The model under review builds one solid part; all positions refer to its coordinate system, in mm. Face numbers are marked on the shaded views. A direction names the side the tool comes from. Coordinates: 2 decimals unless noted, no trailing zeros. Write each loop counter-clockwise with the first axis right and the second up, starting at its lowest first coordinate (ties: lowest second). Pieces come first, ordered by that corner, then holes. Notation, with made-up numbers: (42, -26) - (84, -26) arc R18 ccw to (84, 6) - close; hole circle Ø5 at (29, 2). An arc over 180 degrees is marked (long way). Use one line per item in the form item = value. Start each with the question number.
```python
from build123d import *

# Parameters (mm, degrees)
CROQUIS3_W              = 44
CROQUIS3_H              = 60.5
SALIENTE_EXTRUIR1_DEPTH = 2
SALIENTE_EXTRUIR2_DEPTH = 19
CROQUIS5_W              = 3
CROQUIS5_H              = 13
SALIENTE_EXTRUIR3_DEPTH = 5
CROQUIS6_W              = 40
CROQUIS6_H              = 56.5
CROQUIS6_W_2            = 38
CROQUIS6_H_2            = 54.5
CORTAR_EXTRUIR1_DEPTH   = 5
SALIENTE_EXTRUIR4_DEPTH = 15
REDONDEO1_R             = 2
CORTAR_EXTRUIR4_DEPTH   = 10
CROQUIS9_R              = 1.6
CORTAR_EXTRUIR5_DEPTH   = 10


with BuildPart() as part:
    # Croquis3 → Saliente-Extruir1 (new body)
    with BuildSketch(Plane(origin=(0, 0, 0), x_dir=(1, 0, 0), z_dir=(0, 1, 0))):
        with Locations((0, 16.480436564)):
            Rectangle(CROQUIS3_W, CROQUIS3_H)
    extrude(amount=SALIENTE_EXTRUIR1_DEPTH)

    # Croquis4 → Saliente-Extruir2 (add)
    with BuildSketch(Plane(origin=(0, 2, 0), x_dir=(1, 0, 0), z_dir=(0, 1, 0))):
        Polygon((-22, -13.769563436), (22, -13.769563436), (22, 46.730436564), (-22, 46.730436564), (-22, 14.730436564), (-19, 14.730436564), (-19, 43.730436564), (19, 43.730436564), (19, -10.769563436), (-19, -10.769563436), (-19, 1.730436564), (-22, 1.730436564), align=None)
    extrude(amount=SALIENTE_EXTRUIR2_DEPTH)

    # Croquis5 → Saliente-Extruir3 (add)
    with BuildSketch(Plane(origin=(0, 2, 0), x_dir=(1, 0, 0), z_dir=(0, 1, 0))):
        with Locations((-20.5, 8.230436564)):
            Rectangle(CROQUIS5_W, CROQUIS5_H)
    extrude(amount=SALIENTE_EXTRUIR3_DEPTH)

    # Croquis6 → Cortar-Extruir1 (cut)
    with BuildSketch(Plane(origin=(0, 21, 0), x_dir=(1, 0, 0), z_dir=(0, 1, 0))):
        with Locations((0, 16.480436564)):
            Rectangle(CROQUIS6_W, CROQUIS6_H)
        with Locations((0, 16.480436564)):
            Rectangle(CROQUIS6_W_2, CROQUIS6_H_2, mode=Mode.SUBTRACT)
    extrude(amount=-CORTAR_EXTRUIR1_DEPTH, mode=Mode.SUBTRACT)

    # Croquis7 → Saliente-Extruir4 (add)
    with BuildSketch(Plane(origin=(0, 21, 0), x_dir=(1, 0, 0), z_dir=(0, 1, 0))):
        Polygon((-22, -7.269563436), (-22, -6.869563436), (-22.8, -6.069563436), (-22.8, -8.469563436), (-22, -7.669563436), align=None)
        Polygon((-22, 24.130436564), (-22, 23.730436564), (-22, 23.330436564), (-22.8, 22.530436564), (-22.8, 24.930436564), align=None)
    extrude(amount=-SALIENTE_EXTRUIR4_DEPTH)

    # Redondeo1
    # the kernel refuses this fillet: 2 mm, written as the material it adds along each edge
    with BuildSketch(Plane(origin=(-22, 6, 11.669563436), x_dir=(0, -1, 0), z_dir=(0, 0, -1))) as redondeo1_piece_1_section:
        with BuildLine():
            CenterArc((1.6, 2), REDONDEO1_R, 216.869897646, 53.130102354)
            Line((0, 0.8), (-0.032, 0.776))
            ThreePointArc((-0.032, 0.776), (-0.04, 0.4), (-0.04, 0))
            Line((-0.04, 0), (0, -0.04))
            Line((0, -0.04), (1.6, -0.04))
            Line((1.6, -0.04), (1.6, 0))
        make_face()
    redondeo1_piece_1 = extrude(amount=8.8, mode=Mode.PRIVATE)
    redondeo1_piece_1 = split(redondeo1_piece_1, bisect_by=Plane(origin=(-21.934112323, 5.657693128, 7.603675758), z_dir=(-0.7071067811865467, 0, -0.7071067811865483)), keep=Keep.TOP, mode=Mode.PRIVATE)
    redondeo1_piece_1 = split(redondeo1_piece_1, bisect_by=Plane(origin=(-21.934112323, 5.657693128, 6.935451113), z_dir=(-0.7071067811865467, 0, 0.7071067811865483)), keep=Keep.TOP, mode=Mode.PRIVATE)
    add(redondeo1_piece_1)
    with BuildSketch(Plane(origin=(-22, 6, -19.330436564), x_dir=(0, -1, 0), z_dir=(0, 0, -1))) as redondeo1_piece_2_section:
        with BuildLine():
            CenterArc((1.6, 2), REDONDEO1_R, 216.869897646, 53.130102354)
            Line((0, 0.8), (-0.032, 0.776))
            ThreePointArc((-0.032, 0.776), (-0.04, 0.4), (-0.04, 0))
            Line((-0.04, 0), (0, -0.04))
            Line((0, -0.04), (1.6, -0.04))
            Line((1.6, -0.04), (1.6, 0))
        make_face()
    redondeo1_piece_2 = extrude(amount=8.8, mode=Mode.PRIVATE)
    redondeo1_piece_2 = split(redondeo1_piece_2, bisect_by=Plane(origin=(-21.934112323, 5.657693128, -23.396324242), z_dir=(-0.707106781186546, 0, -0.7071067811865491)), keep=Keep.TOP, mode=Mode.PRIVATE)
    redondeo1_piece_2 = split(redondeo1_piece_2, bisect_by=Plane(origin=(-21.934112323, 5.657693128, -24.064548887), z_dir=(-0.7071067811865476, 0, 0.7071067811865476)), keep=Keep.TOP, mode=Mode.PRIVATE)
    add(redondeo1_piece_2)

    # Croquis8 → Cortar-Extruir4 (cut)
    with BuildSketch(Plane(origin=(22, 0, 0), x_dir=(0, 0, -1), z_dir=(1, 0, 0))):
        with BuildLine():
            Line((15.097928983, 8.744612484), (15.130436564, 8.814093536))
            Line((15.130436564, 8.814093536), (15.130436564, 15.185906464))
            ThreePointArc((15.130436564, 15.185906464), (8.230436564, 19.6), (1.330436564, 15.185906464))
            Line((1.330436564, 15.185906464), (1.330436564, 8.814093536))
            ThreePointArc((1.330436564, 8.814093536), (8.192081775, 4.400096783), (15.097928983, 8.744612484))
        make_face()
    extrude(amount=-CORTAR_EXTRUIR4_DEPTH, mode=Mode.SUBTRACT)

    # Croquis9 → Cortar-Extruir5 (cut)
    with BuildSketch(Plane.ZY.offset(22)):
        with Locations((-18.980436564, 13)):
            Circle(CROQUIS9_R)
        with Locations((2.519563436, 13)):
            Circle(CROQUIS9_R)
    extrude(amount=-CORTAR_EXTRUIR5_DEPTH, mode=Mode.SUBTRACT)


solid = part.part
```
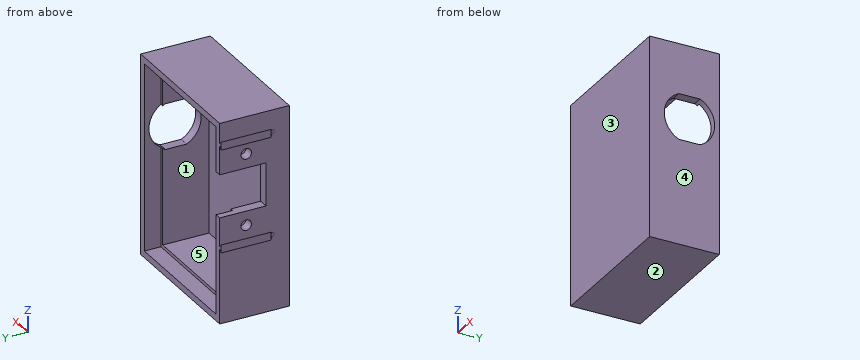
1. The part is to be moulded in two halves that separate along X. For the marked faces 3, 4 and 5, say which applies: released by +X, released by -X, zero draft, split by the parting line, or undercut.
2. Take a section at A-A (y = 10.5). State the section outline as (x, z) points, plus the area to 3 significant figures.
3. Take a section at C-C (x = 13). State the section outline as (y, z) points.
4. For L1, parallel to X at y = 14.75, z = 0.5; L2, parallel to X at y = 19.75, z = -31.5; L3, parallel to Z at x = 11, y = 17, list the stretches that pass through material, from the lowest coordinate up.
5. For the marked faces 1 and 2, list the 3-axis set-ups (+Z, -Z, +X, -X, +Y, -Y) from which the entire face can be reached by the end or side of a thin tool; tool diameter is ignored.
6. Take a section at B-B (z = 2). State the section outline as (x, y) points.
7. For P1, Ø11, axis at x = 6.5, z = 1.5, coming from the +Y side; P2, Ø1.5, axis at x = -20, z = -10, coming from the +Y side; P3, Ø3, axis at y = 11.5, z = -2, coming from the -X side, all flat-tipped, find the tip position at first contact; note any pin that passes through.
Returned:
q1.face_3 = zero draft
q1.face_4 = released by +X
q1.face_5 = undercut
q2.outline = (-22.8, -24.93) - (-22, -24.13) - (-22, -46.73) - (22, -46.73) - (22, -15.13) - (19, -15.13) - (19, -43.73) - (-19, -43.73) - (-19, -14.73) - (-22, -14.73) - (-22, -23.33) - (-22.8, -22.53) - close; (-22.8, 6.07) - (-22, 6.87) - (-22, -1.73) - (-19, -1.73) - (-19, 10.77) - (19, 10.77) - (19, -1.33) - (22, -1.33) - (22, 13.77) - (-22, 13.77) - (-22, 7.67) - (-22.8, 8.47) - close
q2.area = 513 mm²
q3.outline = (0, -46.73) - (21, -46.73) - (21, -44.73) - (16, -44.73) - (16, -43.73) - (2, -43.73) - (2, 10.77) - (16, 10.77) - (16, 11.77) - (21, 11.77) - (21, 13.77) - (0, 13.77) - close
q4.L1 = -22 to -19, 19 to 22
q4.L2 = -22 to -20, 20 to 22
q4.L3 = -46.73 to -44.73, 11.77 to 13.77
q5.face_1 = +Y
q5.face_2 = -Z, +X, -X, +Y, -Y
q6.outline = (-22, 0) - (22, 0) - (22, 21) - (20, 21) - (20, 16) - (19, 16) - (19, 2) - (-19, 2) - (-19, 11.49) - (-22, 11.49) - close; (-22, 14.51) - (-19, 14.51) - (-19, 16) - (-20, 16) - (-20, 21) - (-22, 21) - close
q7.P1 = 2
q7.P2 = 7
q7.P3 = -22
